from build123d import *

# Parameters (mm, degrees)
F0_R     = 39.76573
F0_R_2   = 18.191508
F1_DEPTH = 179.832
F4_DEPTH = 50.8
F5_DEPTH = 50.8


with BuildPart() as f1:
    # F0 (on Front) → F1 (new body)
    with BuildSketch(Plane.XZ):
        Circle(F0_R)
        Circle(F0_R_2, mode=Mode.SUBTRACT)
    extrude(amount=F1_DEPTH)

    # F3 (on face) → F4 (join)
    with BuildSketch(Plane(origin=(0, 0, 0), x_dir=(-1, 0, 0), z_dir=(0, 1, 0))):
        with BuildLine():
            Line((-39.76573, 99.41814), (-39.76573, 0))
            ThreePointArc((-39.76573, 0), (0, 39.76573), (39.76573, 0))
            Line((39.76573, 0), (39.76573, 99.41814))
            Line((39.76573, 99.41814), (21.730875, 99.41814))
            ThreePointArc((21.730875, 99.41814), (0, 77.687265), (-21.730875, 99.41814))
            Line((-21.730875, 99.41814), (-39.76573, 99.41814))
        make_face()
        with BuildLine():
            ThreePointArc((39.76573, 99.41814), (0, 139.18387), (-39.76573, 99.41814))
            Line((-39.76573, 99.41814), (-21.730875, 99.41814))
            ThreePointArc((-21.730875, 99.41814), (0, 121.149015), (21.730875, 99.41814))
            Line((21.730875, 99.41814), (39.76573, 99.41814))
        make_face()
    extrude(amount=-F4_DEPTH)

    # F2 (on face) → F5 (join)
    with BuildSketch(Plane.XZ.offset(179.832)):
        with BuildLine():
            Line((-39.76573, 99.418327), (-39.76573, 0))
            ThreePointArc((-39.76573, 0), (0, 39.76573), (39.76573, 0))
            Line((39.76573, 0), (39.76573, 99.418327))
            Line((39.76573, 99.418327), (21.730875, 99.418327))
            ThreePointArc((21.730875, 99.418327), (0, 77.687452), (-21.730875, 99.418327))
            Line((-21.730875, 99.418327), (-39.76573, 99.418327))
        make_face()
        with BuildLine():
            ThreePointArc((39.76573, 99.418327), (0, 139.184057), (-39.76573, 99.418327))
            Line((-39.76573, 99.418327), (-21.730875, 99.418327))
            ThreePointArc((-21.730875, 99.418327), (0, 121.149202), (21.730875, 99.418327))
            Line((21.730875, 99.418327), (39.76573, 99.418327))
        make_face()
    extrude(amount=-F5_DEPTH)


solid = f1.part
Part model, mm, in its own coordinate system. Give positions to 0.01 mm unless a question says otherwise; leave off trailing zeros. Write each loop counter-clockwise with the first axis right and the second up, starting at its lowest first coordinate (ties: lowest second). Pieces come first, ordered by that corner, then holes.
1) Two-plate mould, pull along Z, no slides. Class faces 1 (the face through (18.35, -88.66, -35.28)), 2 (the face through (4.7, -154.8, 78.2)), 3 (the face through (-39.766, -25, 49)), 4 (the face through (-0.874, -25.044, 139.174)): released by +Z, released by -Z, zero draft, split by the parting line, or undercut.
Resolved:
face 1: split by the parting line
face 2: undercut
face 3: zero draft
face 4: released by +Z
2) Cut at A-A on x = 0. Write the cut outline in (y, z).
Resolved:
outline: (-179.83, -39.77) - (0, -39.77) - (0, -18.19) - (-179.83, -18.19) - close; (-179.83, 18.19) - (0, 18.19) - (0, 77.69) - (-50.8, 77.69) - (-50.8, 39.77) - (-129.03, 39.77) - (-129.03, 77.69) - (-179.83, 77.69) - close; (-179.83, 121.15) - (-129.03, 121.15) - (-129.03, 139.18) - (-179.83, 139.18) - close; (-50.8, 121.15) - (0, 121.15) - (0, 139.18) - (-50.8, 139.18) - close
3) Cut at D-D on z = 118. Write the cut outline in (x, y).
Resolved:
outline: (-35.16, -179.83) - (-11.27, -179.83) - (-11.27, -129.03) - (-35.16, -129.03) - close; (-35.16, -50.8) - (-11.27, -50.8) - (-11.27, 0) - (-35.16, 0) - close; (11.27, -179.83) - (35.16, -179.83) - (35.16, -129.03) - (11.27, -129.03) - close; (11.27, -50.8) - (35.16, -50.8) - (35.16, 0) - (11.27, 0) - close
4) Probe L1, parallel to Z at x = 0, y = -17; L2, parallel to Y at x = 10, z = 69.5; L3, parallel to Z at x = 0, y = -96. List the from-to ranges inside material, lowest first.
Resolved:
L1: z = -39.77 to -18.19, 18.19 to 77.69, 121.15 to 139.18
L2: y = -179.83 to -129.03, -50.8 to 0
L3: z = -39.77 to -18.19, 18.19 to 39.77
5) Cut at C-C on y = -137. Write the cut outline in (x, z).
Resolved:
outline: (-39.77, 0) arc R39.77 ccw to (39.77, 0) - (39.77, 99.42) arc R39.77 ccw to (-39.77, 99.42) - close; hole circle Ø43.46 at (0, 99.42); hole circle Ø36.38 at (0, 0)
6) Cut at B-B on z = 70.5. Write the cut outline in (x, y).
Resolved:
outline: (-39.77, -179.83) - (39.77, -179.83) - (39.77, -129.03) - (-39.77, -129.03) - close; (-39.77, -50.8) - (39.77, -50.8) - (39.77, 0) - (-39.77, 0) - close
7) Pin check, flat tips, straight feed: pin 1 (8 mm diameter, centred on x = 24.5, y = -33, fed in from +Z); pin 2 (10 mm diameter, centred on x = -23, y = -129.5, fed in from -Z); pin 3 (3 mm diameter, centred on x = 5, y = -90, fed in from +Z). Stop position of each tip, or through.
Resolved:
pin 1: stops at z = 133.49
pin 2: stops at z = -35.46
pin 3: stops at z = 39.61
